Input: part model. Units: mm. Frame: model coordinates. Face numbers are marked on the shaded views. A direction names the side the tool comes from. Round coordinates to 2 decimals unless told otherwise and drop trailing zeros. Loops run counter-clockwise (first coordinate to the right, second up) from the corner with the lowest first, then second, coordinate; pieces in that order, holes last. Notation, with made-up numbers: M 34.25,-12.5 L 91.25,-12.5 A26 ccw 91.25,8.5 Z; hole C 20,-36 d3. An arc over 180 degrees is marked long. Use one line per item in the form item = value. Start each with the question number.
Q1. Section query A-A, the plane y = 0. Output: boundary loops of the cut face in (x, z) (3 decimals).
Q2. Section query C-C, the plane z = 28.5. Output: boundary loops of the cut face in (x, y) (3 decimals), and give its area (3 significant figures).
Q3. Section query B-B, the plane x = 0. Output: boundary loops of the cut face in (y, z) (3 decimals).
Q4. Access query for the marked faces 1, 2 and 3. Directions: +Z, -Z, +X, -X, +Y, -Y. A direction counts if a zero-diameter tool reaches every point of the face in a straight line with its end or side. Return the directions, or none.
Q5. Section query D-D, the plane z = 5. Output: boundary loops of the cut face in (x, y) (3 decimals), and give its area (3 significant figures).
Q6. First-contact query: P1, Ø1.8, axis at x = 1.5, z = 40, coming from the +Y side (3 decimals); P2, Ø1.5, axis at y = -1.5, z = 25.5, coming from the -X side; P3, Ø0.5, axis at x = -1.5, y = 0, coming from the +Z side. Flat tips, straight axial feed; report the tip coordinate or a pass-through.
Q7. Ray query, line 1 along Z through (x, y) = (3, -0.5); line 2 along Z through (x, y) = (0.5, -0.5); line 3 along Z through (x, y) = (2.25, 1.75). Return the intervals inside material, ascending.
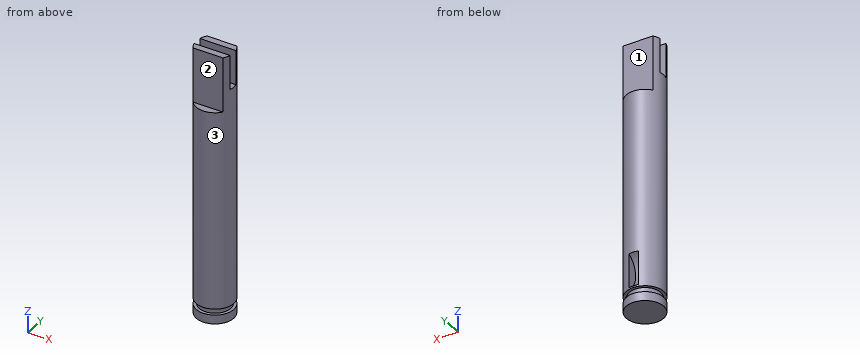
```python
from build123d import *

# Parameters (mm, degrees)
SKETCH1_R           = 3.175
EXTRUDE1_DEPTH      = 42.926
SKETCH4_R           = 3.175
EXTRUDE2_DEPTH      = 0.79375
EXTRUDE2_DEPTH_BACK = 0.79375
SKETCH5_R           = 3.175
EXTRUDE3_DEPTH      = 2.54
SKETCH6_OUTSIDE_W   = 17.618
SKETCH6_OUTSIDE_H   = 17.618
SKETCH6_OUTSIDE_R   = 2.667
EXTRUDE4_DEPTH      = 1.016
EXTRUDE5_DEPTH      = 4.1750001
EXTRUDE5_DEPTH_BACK = 4.1750001
EXTRUDE6_DEPTH      = 4.1750001


with BuildPart() as part:
    # Sketch1 → Extrude1 (new body)
    with BuildSketch(Plane.XY):
        Circle(SKETCH1_R)
    extrude(amount=EXTRUDE1_DEPTH)

    # Sketch4 → Extrude2 (cut, two sides)
    with BuildSketch(Plane(origin=(0, 0, 0), x_dir=(0, 0, -1), z_dir=(1, 0, 0))) as extrude2_sk:
        with Locations((-3.175, 4.445)):
            Circle(SKETCH4_R)
    extrude(amount=EXTRUDE2_DEPTH, mode=Mode.SUBTRACT)
    extrude(extrude2_sk.sketch, amount=-EXTRUDE2_DEPTH_BACK, mode=Mode.SUBTRACT)

    # Sketch5 → Extrude3 (add)
    with BuildSketch(Plane(origin=(0, 0, 0), x_dir=(-1, 0, 0), z_dir=(0, 0, -1))):
        Circle(SKETCH5_R)
    extrude(amount=EXTRUDE3_DEPTH)

    # Sketch6 outside → Extrude4 (cut)
    with BuildSketch(Plane.XY):
        Rectangle(SKETCH6_OUTSIDE_W, SKETCH6_OUTSIDE_H)
        Circle(SKETCH6_OUTSIDE_R, mode=Mode.SUBTRACT)
    extrude(amount=-EXTRUDE4_DEPTH, mode=Mode.SUBTRACT)

    # Sketch7 → Extrude5 (cut, two sides)
    with BuildSketch(Plane(origin=(0, 0, 0), x_dir=(0, 0, -1), z_dir=(1, 0, 0))) as extrude5_sk:
        Polygon((-42.926, 0), (-42.926, 0.7874), (-37.084, 0.7874), (-37.084, 0), (-37.084, -0.7874), (-42.926, -0.7874), align=None)
    extrude(amount=EXTRUDE5_DEPTH, mode=Mode.SUBTRACT)
    extrude(extrude5_sk.sketch, amount=-EXTRUDE5_DEPTH_BACK, mode=Mode.SUBTRACT)

    # Sketch8 → Extrude6 (cut, symmetric)
    with BuildSketch(Plane(origin=(0, 0, 0), x_dir=(0, 0, -1), z_dir=(1, 0, 0))):
        Polygon((-42.926, 1.905), (-40.005, 1.905), (-33.655, 1.905), (-33.655, 3.175), (-42.926, 3.175), align=None)
    extrude6 = extrude(amount=EXTRUDE6_DEPTH, both=True, mode=Mode.SUBTRACT)

    # Mirror1: Extrude6 across plane
    add(extrude6.mirror(Plane.ZX), mode=Mode.SUBTRACT)


solid = part.part
```
Results found:
q1.outline = M -3.175,-2.54 L 3.175,-2.54 L 3.175,-1.016 L 2.667,-1.016 L 2.667,0 L 3.175,0 L 3.175,37.084 L -3.175,37.084 L -3.175,0 L -2.667,0 L -2.667,-1.016 L -3.175,-1.016 Z
q2.outline = C 0,0 d6.35
q2.area = 31.7 mm²
q3.outline = M -3.175,-2.54 L 3.175,-2.54 L 3.175,-1.016 L 2.667,-1.016 L 2.667,0 L 3.175,0 L 3.175,0.265 A3.175 cw 3.175,6.085 L 3.175,33.655 L 1.905,33.655 L 1.905,42.926 L 0.787,42.926 L 0.787,37.084 L -0.787,37.084 L -0.787,42.926 L -1.905,42.926 L -1.905,33.655 L -3.175,33.655 L -3.175,0 L -2.667,0 L -2.667,-1.016 L -3.175,-1.016 Z
q4.face_1 = +Z, +X, -X, +Y
q4.face_2 = +Z, +X, -X, -Y
q4.face_3 = +Z, -Z
q5.outline = M -0.794,1.847 L -0.794,3.074 A3.175 ccw long 0.794,3.074 L 0.794,1.847 Z
q5.area = 29.6 mm²
q6.P1 = 1.905
q6.P2 = -3.09
q6.P3 = 37.08
q7.line_1 = -2.54 to -1.02, 0 to 37.08
q7.line_2 = -2.54 to 37.08
q7.line_3 = -2.54 to -1.02, 0 to 42.93
